Study the drawing (mm; zero at the part's minimum x, y, z) and answer. A direction names the side the tool comes from. Coordinates: 2 decimals unless noted, no trailing zeros. Loops run counter-clockwise (first coordinate to the right, second up) from the corner with the lowest first, then second, coordinate; pieces in that order, holes last.
Q1. Flat-ended cylindrical pins translate along their axes: P1, Ø12, axis at y = 74.5, z = 32, coming from the -X side; P2, Ø9, axis at x = 39.5, y = 58, coming from the -Z side; P3, Ø5.5, axis at x = 9.5, z = 34, coming from the +Y side; P4, Ø4, axis at y = 50, z = 81.5, coming from the -X side. Find the tip coordinate at first contact, or state that the pin passes through.
Q2. Section B-B (x = 37) is taken. Give the vertices of the cut face in (y, z).
Q3. Section A-A (z = 32) is taken. Give the vertices of the cut face in (x, y), then the cut area to 3 significant figures.
Q4. Which of the six approach directions +Z, -Z, +X, -X, +Y, -Y give full straight-line access (tool end or side, diameter ignored) to the marked faces 5, 6 and 7?
Q5. Section C-C (y = 40) is taken. Give the vertices of the cut face in (x, z), then the cut area to 3 significant figures.
Q6. Straight lines are drawn through the part: line 1 (Z direction, x = 43, y = 66); line 2 (Y direction, x = 13, z = 50); line 3 (X direction, y = 49.5, z = 31). For each, find the intervals that lie inside material, in ascending order.
Q7. The mould has two halves that part along Y. Classify the marked faces 1, 2, 3 and 4: pulls with the +Y half, pulls with the -Y half, needs draft (parallel to the pull), parting line crosses it, or undercut.
Q8. Section D-D (x = 30) is taken. Give the vertices of the cut face in (y, z).
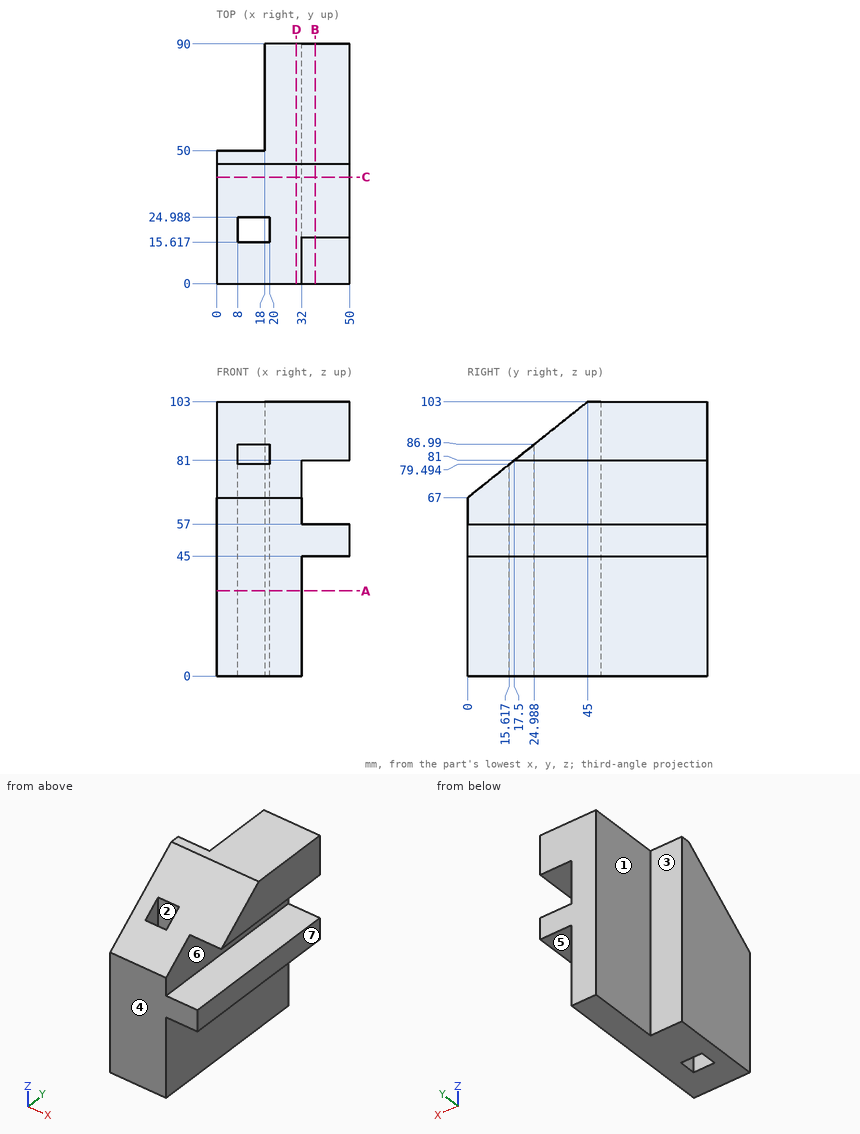
Numbers:
1. P1: stops at x = 18
1. P2: stops at z = 45
1. P3: stops at y = 50
1. P4: stops at x = 0
2. outline: (0, 45) - (90, 45) - (90, 57) - (0, 57) - close; (17.5, 81) - (90, 81) - (90, 103) - (45, 103) - close
3. outline: (0, 0) - (32, 0) - (32, 90) - (18, 90) - (18, 50) - (0, 50) - close; hole (8, 15.62) - (20, 15.62) - (20, 24.99) - (8, 24.99) - close
3. area: 2,050 mm2
4. face 5: -Z, +X, +Y, -Y
4. face 6: +X, +Y, -Y
4. face 7: +Z, -Z, +X, +Y, -Y
5. outline: (0, 0) - (32, 0) - (32, 45) - (50, 45) - (50, 57) - (32, 57) - (32, 81) - (50, 81) - (50, 99) - (0, 99) - close
5. area: 3,710 mm2
6. line 1: z = 45 to 57, 81 to 103
6. line 2: y = 0 to 15.62, 24.99 to 50
6. line 3: x = 0 to 32
7. face 1: needs draft
7. face 2: undercut
7. face 3: pulls with the +Y half
7. face 4: pulls with the -Y half
8. outline: (0, 0) - (90, 0) - (90, 103) - (45, 103) - (0, 67) - close
